Geometry check sheet. Reference: drawing and pictorial views, mm from the part's lowest x, y, z. Round coordinates to 2 decimals unless told otherwise and drop trailing zeros. Order: outer loops, then holes, each group sorted by start corner. A loop starts at its lowest first (then second) coordinate and runs counter-clockwise, first axis right, second up. Notation, with made-up numbers: (-2.75, 3.5) -> (37.25, 3.5) arc R20 cw to (37.25, 34.5) -> close; hole circle Ø3 at (64.5, 49). An arc over 180 degrees is marked (long way). Return JSON: item names as keys, results as strings. Group by question number.
1) Section check C-C on z = 3.75. Enter the section's corners in (x, y), plus the area to 3 significant figures.
2) Draft check along X on the marked faces 1, 2 and 3. Enter one of: pulls with the +X half, pulls with the -X half, needs draft (parallel to the pull), parting line crosses it, or undercut.
3) Section check A-A on x = 17. Enter the section's corners in (y, z), plus the area to 4 significant figures.
4) Depth check by flat-ended pin: pin 1 (1 mm diameter, centred on x = 23, z = 3.5, fed in from -Y) (3 decimals); pin 2 (17.5 mm diameter, centred on x = 22, y = 13, fed in from -Z); pin 3 (5 mm diameter, centred on x = 15.5, z = 7, fed in from -Y); pin 4 (17.5 mm diameter, centred on x = 17, y = 17, fed in from -Z). Enter the tip coordinate at first touch or a pass-through.
5) Scan lines: L1, parallel to Y at x = 17, z = 7.25; L2, parallel to Z at x = 18, y = 3. Record each from-to range of solid material in increasing order.
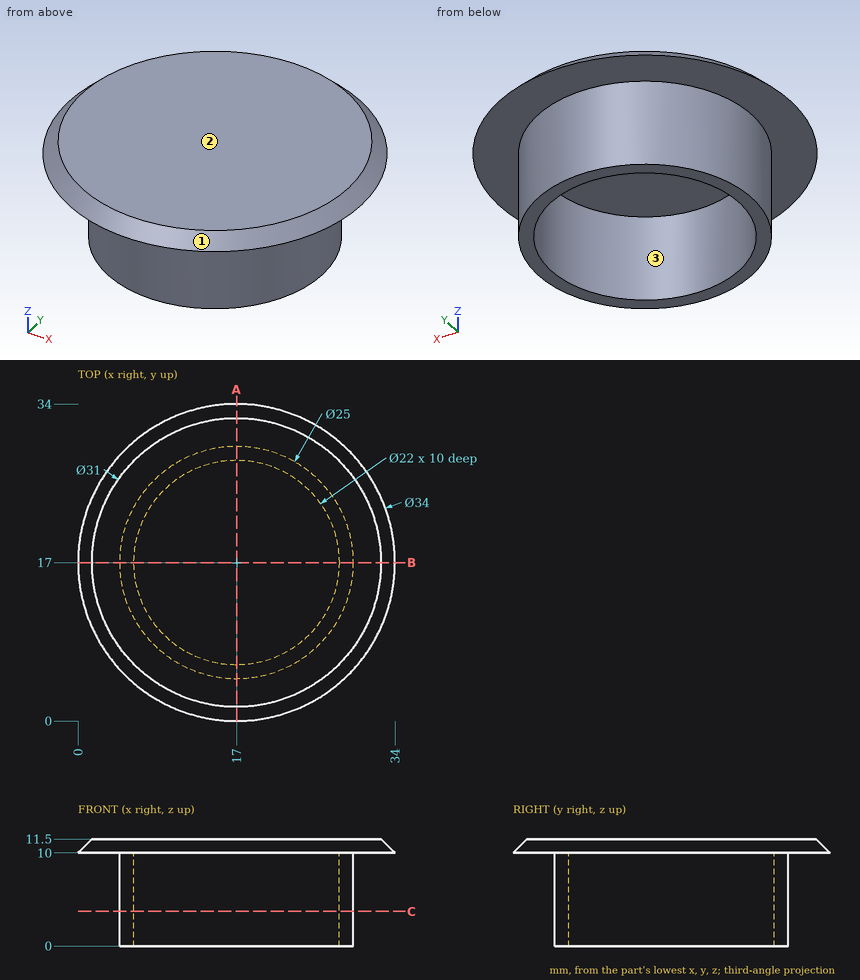
Check result:
{
 "1": {"outline": "circle Ø25 at (17, 17); hole circle Ø22 at (17, 17)", "area": "111 mm^2"},
 "2": {"face 1": "parting line crosses it", "face 2": "needs draft", "face 3": "undercut"},
 "3": {"outline": "(0, 10) -> (4.5, 10) -> (4.5, 0) -> (6, 0) -> (6, 10) -> (28, 10) -> (28, 0) -> (29.5, 0) -> (29.5, 10) -> (34, 10) -> (32.5, 11.5) -> (1.5, 11.5) -> close", "area": "78.75 mm^2"},
 "4": {"pin 1": "y = 5.775", "pin 2": "z = 0", "pin 3": "y = 4.5", "pin 4": "z = 10"},
 "5": {"L1": "4.5 to 6, 28 to 29.5", "L2": "10 to 11.5"}
}
